Design review of the part built by this model. Coordinates are the model's own, in mm. Round coordinates to 2 decimals unless told otherwise and drop trailing zeros. Order: outer loops, then holes, each group sorted by start corner. A loop starts at its lowest first (then second) coordinate and runs counter-clockwise, first axis right, second up.
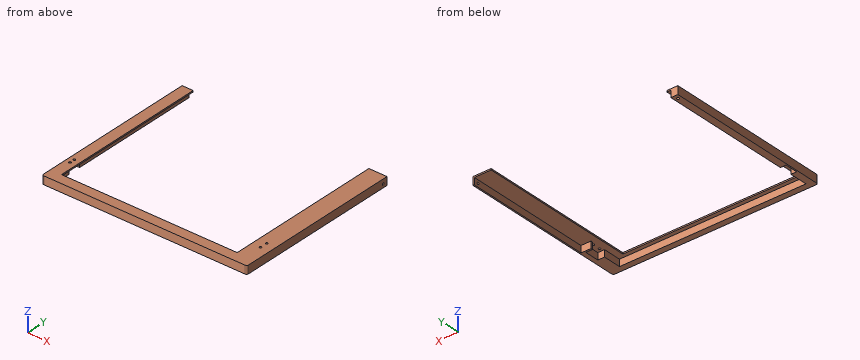
Autodesk Inventor part; units mm, degrees
ref_plane "YZ Plane" through (0, 0, 0) normal (1, 0, 0) x (0, 1, 0)
ref_plane "XZ Plane" through (0, 0, 0) normal (0, 1, 0) x (-1, 0, 0)
ref_plane "XY Plane" through (0, 0, 0) normal (0, 0, 1) x (1, 0, 0)
sketch "Boceto1" plane through (0, 0, 0) normal (0, 0, 1) x (1, 0, 0)
  circle A0 centre (100.65, -156.7) radius 1.65
  circle A1 centre (100.65, -148.3) radius 1.65
  circle A2 centre (100.65, 156.7) radius 1.65
  circle A3 centre (100.65, 148.3) radius 1.65
  line L0 (97.75, 145) -> (105.25, 145)
  line L1 (105.25, 145) -> (105.25, 160)
  line L2 (105.25, 160) -> (97.75, 160)
  line L3 (97.75, 160) -> (97.75, 180)
  line L4 (97.75, 180) -> (-109, 180)
  line L5 (-109, 160) -> (-115.3, 160)
  line L6 (-109, -160) -> (-109, -180)
  line L7 (-115.3, 146.9) -> (-109, 146.9)
  line L8 (-109, -146.9) -> (-115.3, -146.9)
  line L9 (-109, 180) -> (-109, 160)
  line L10 (-115.3, -160) -> (-109, -160)
  line L11 (-109, -180) -> (97.75, -180)
  line L12 (97.75, -180) -> (97.75, -160)
  line L13 (97.75, -160) -> (105.25, -160)
  line L14 (105.25, -160) -> (105.25, -145)
  line L15 (105.25, -145) -> (97.75, -145)
  line L16 (97.75, -145) -> (97.75, -142)
  line L17 (97.75, -142) -> (109, -142)
  line L18 (109, -142) -> (109, 142)
  line L19 (109, 142) -> (97.75, 142)
  line L20 (97.75, 142) -> (97.75, 145)
  line L21 (109, 180) -> (97.75, 180)
  line L22 (-109, -160) -> (-109, -180)
  line L23 (-109, -180) -> (-102.7, -180)
  line L24 (-109, -180) -> (109, -180)
  line L25 (109, -180) -> (109, 180)
  line L26 (109, 180) -> (-109, 180)
  line L27 (111, 142) -> (111, 180)
  line L28 (109, 182) -> (97.75, 182)
  line L29 (-109, -182) -> (-102.7, -182)
  line L30 (-111, -182) -> (111, -182)
  line L31 (111, -182) -> (111, 182)
  line L32 (111, 182) -> (-111, 182)
  circle A4 centre (-111.9, -156.3) radius 1.2
  circle A5 centre (-111.9, -150.6) radius 1.2
  circle A6 centre (-111.9, 156.3) radius 1.2
  circle A7 centre (-111.9, 150.6) radius 1.2
  line L33 (-115.3, 160) -> (-115.3, 146.9)
  line L34 (-109, 146.9) -> (-109, -146.9)
  line L35 (-115.3, -146.9) -> (-115.3, -160)
  line L36 (-109, 180) -> (-115.3, 180)
  line L37 (-109, -180) -> (-115.3, -180)
  line L38 (-115.3, 180) -> (109, 180)
  line L39 (109, 180) -> (109, -180)
  line L40 (109, -180) -> (-115.3, -180)
  line L41 (-115.3, -180) -> (-115.3, 180)
  line L42 (-117.3, 180) -> (-117.3, -182)
  line L43 (-117.3, -182) -> (109, -182)
  line L44 (-115.3, 182) -> (111, 182)
  line L45 (111, 182) -> (111, -180)
  line L46 (-117.3, 180) -> (-117.3, 182)
  line L47 (-117.3, 182) -> (-115.3, 182)
  point P0 (0, 0)
  dimension "d1" = 2
  dimension "d3" = 2
  dimension "d20" = 2
  dimension "d21" = 2
extrude "Extrusión1" add sketch "Boceto1" against normal blind 7.5 contours L0 L1 L2 L3 L21 L25 L19 L20 | L25 L24 L12 L13 L14 L15 L16 L17 | L9 L5 L41 L36 | L37 L41 L10 L6 | L7 L34 L8 L41 | L31 L30 L29 L43 L42 L46 L47 L44 L32 L28 L27
sketch "Boceto2" plane through (0, 0, 0) normal (0, 0, 1) x (1, 0, 0)
  line L0 (-117.3, -182) -> (111, -182)
  line L1 (111, -182) -> (111, 182)
  line L2 (111, 182) -> (-117.3, 182)
  line L3 (90.8, 170.8) -> (90.8, -176)
  line L4 (90.8, 170.8) -> (90.8, -176)
  line L5 (-19.4789, -176) -> (90.8, -176)
  line L6 (90.8, -176) -> (-99.7, -176)
  line L7 (-99.7, -176) -> (-99.7, 170.8)
  line L8 (-99.7, 170.8) -> (90.8, 170.8)
  line L9 (-117.3, 182) -> (-117.3, -182)
  line L10 (-105.5008, -176) -> (-99.7, -176)
  line L11 (-99.7, 170.8) -> (-105.5008, 170.8)
  line L12 (-109, 160) -> (-109, 180)
  line L13 (-109, 170.8) -> (-105, 170.8)
  line L14 (-105, 170.8) -> (-105, -176)
  point P0 (0, 0)
  dimension "d33" = 4
extrude "Extrusión2" add sketch "Boceto2" along normal blind 1.5
sketch "Boceto3" plane through (-111, -182, -7.5) normal (0, -1, 0) x (1, 0, 0)
  line L0 (222, 0) -> (-6.3, 0)
  line L1 (222, 0) -> (222, 9)
  line L2 (-6.3, 9) -> (222, 9)
  line L3 (-6.3, 0) -> (-6.3, 9)
  point P0 (111, 7.5)
extrude "Extrusión3" add sketch "Boceto3" along normal blind 5.2
sketch "Boceto5" plane through (0, 0, 1.5) normal (0, 0, 1) x (1, 0, 0)
  circle A0 centre (100.65, -156.7) radius 1.65
  circle A1 centre (100.65, -148.3) radius 1.65
  circle A2 centre (100.65, 156.7) radius 1.65
  circle A3 centre (100.65, 148.3) radius 1.65
  line L0 (97.75, 145) -> (105.25, 145)
  line L1 (105.25, 145) -> (105.25, 160)
  line L2 (105.25, 160) -> (97.75, 160)
  line L3 (97.75, 160) -> (97.75, 180)
  line L4 (97.75, 180) -> (-109, 180)
  line L5 (-109, 160) -> (-115.3, 160)
  line L6 (-109, -160) -> (-109, -180)
  line L7 (-115.3, 146.9) -> (-109, 146.9)
  line L8 (-109, -146.9) -> (-115.3, -146.9)
  line L9 (-109, 180) -> (-109, 160)
  line L10 (-115.3, -160) -> (-109, -160)
  line L11 (-109, -180) -> (97.75, -180)
  line L12 (97.75, -180) -> (97.75, -160)
  line L13 (97.75, -160) -> (105.25, -160)
  line L14 (105.25, -160) -> (105.25, -145)
  line L15 (105.25, -145) -> (97.75, -145)
  line L16 (97.75, -145) -> (97.75, -142)
  line L17 (97.75, -142) -> (109, -142)
  line L18 (109, -142) -> (109, 142)
  line L19 (109, 142) -> (97.75, 142)
  line L20 (97.75, 142) -> (97.75, 145)
  circle A4 centre (-111.9, -156.3) radius 1.2
  circle A5 centre (-111.9, -150.6) radius 1.2
  circle A6 centre (-111.9, 156.3) radius 1.2
  circle A7 centre (-111.9, 150.6) radius 1.2
  line L21 (-115.3, 160) -> (-115.3, 146.9)
  line L22 (-109, 146.9) -> (-109, -146.9)
  line L23 (-115.3, -146.9) -> (-115.3, -160)
  point P0 (0, 0)
hole "Agujero1" at (100.65, 148.3, 1.5) at (100.65, 156.7, 1.5) at (100.65, -156.7, 1.5) at (100.65, -148.3, 1.5) at (-111.9, -156.3, 1.5) at (-111.9, -150.6, 1.5) at (-111.9, 150.6, 1.5) at (-111.9, 156.3, 1.5) direction (0, 0, -1) diameter 2.4 end through all
sketch "Boceto6" plane through (0, 0, -7.5) normal (0, 0, -1) x (-1, 0, 0)
  line L0 (117.3, 182) -> (-111, 182)
  line L1 (-111, 182) -> (-111, -187.2)
  line L2 (117.3, -187.2) -> (-111, -187.2)
  line L3 (117.3, 182) -> (117.3, -187.2)
  line L4 (-97.75, 160) -> (-97.75, 180)
  line L5 (-97.75, 180) -> (109, 180)
  line L6 (109, 180) -> (109, 160)
  line L7 (109, 160) -> (115.3, 160)
  line L8 (115.3, 160) -> (115.3, 146.9)
  line L9 (115.3, 146.9) -> (109, 146.9)
  line L10 (109, 146.9) -> (109, -146.9)
  line L11 (109, -146.9) -> (115.3, -146.9)
  line L12 (115.3, -146.9) -> (115.3, -160)
  line L13 (115.3, -160) -> (109, -160)
  line L14 (109, -160) -> (109, -180)
  line L15 (109, -180) -> (-97.75, -180)
  line L16 (-97.75, -180) -> (-97.75, -160)
  line L17 (-97.75, -160) -> (-105.25, -160)
  line L18 (-105.25, -160) -> (-105.25, -145)
  line L19 (-105.25, -145) -> (-97.75, -145)
  line L20 (-97.75, -145) -> (-97.75, -142)
  line L21 (-97.75, -142) -> (-109, -142)
  line L22 (-109, -142) -> (-109, 142)
  line L23 (-109, 142) -> (-97.75, 142)
  line L24 (-97.75, 142) -> (-97.75, 145)
  line L25 (-97.75, 145) -> (-105.25, 145)
  line L26 (-105.25, 145) -> (-105.25, 160)
  line L27 (-105.25, 160) -> (-97.75, 160)
  line L28 (117.3, 182) -> (117.3, -187.2)
  line L29 (117.3, 182) -> (-111, 182)
  line L30 (-111, 182) -> (-111, -187.2)
  line L31 (117.3, -187.2) -> (-111, -187.2)
  line L32 (109.5, 160.5) -> (109.5, 180.5)
  line L33 (109.5, 180.5) -> (-98.25, 180.5)
  line L34 (-98.25, 180.5) -> (-98.25, 160.5)
  line L35 (-98.25, 160.5) -> (-105.75, 160.5)
  line L36 (-105.75, 160.5) -> (-105.75, 144.5)
  line L37 (-105.75, 144.5) -> (-98.25, 144.5)
  line L38 (-98.25, 144.5) -> (-98.25, 142.5)
  line L39 (-98.25, 142.5) -> (-109.5, 142.5)
  line L40 (-109.5, 142.5) -> (-109.5, -142.5)
  line L41 (-109.5, -142.5) -> (-98.25, -142.5)
  line L42 (-98.25, -142.5) -> (-98.25, -144.5)
  line L43 (-98.25, -144.5) -> (-105.75, -144.5)
  line L44 (-105.75, -144.5) -> (-105.75, -160.5)
  line L45 (-105.75, -160.5) -> (-98.25, -160.5)
  line L46 (-98.25, -160.5) -> (-98.25, -180.5)
  line L47 (-98.25, -180.5) -> (109.5, -180.5)
  line L48 (109.5, -180.5) -> (109.5, -160.5)
  line L49 (109.5, -160.5) -> (115.8, -160.5)
  line L50 (115.8, -160.5) -> (115.8, -146.4)
  line L51 (115.8, -146.4) -> (109.5, -146.4)
  line L52 (109.5, -146.4) -> (109.5, 146.4)
  line L53 (109.5, 146.4) -> (115.8, 146.4)
  line L54 (115.8, 146.4) -> (115.8, 160.5)
  line L55 (115.8, 160.5) -> (109.5, 160.5)
  dimension "d22" = 0.5
extrude "Extrusión4" cut sketch "Boceto6" against normal blind 7.5 contours L55 L54 L53 L52 L51 L50 L49 L48 L47 L46 L45 L44 L43 L42 L41 L40 L39 L38 L37 L36 L35 L34 L33 L32
fillet "Empalme1" radius 2 5 edges at (-117.3, 182, 0.75) (-117.3, 182, -3.75) (111, 182, -3) (111, -187.2, -3) (-117.3, -187.2, -3)
sketch "Boceto7" plane through (0, 0, -7.5) normal (0, 0, -1) x (-1, 0, 0)
  arc A0 (117.3, 7) -> (114.3, 10) centre (114.3, 7) ccw
  line L0 (114.3, 10) -> (100.3, 10)
  arc A1 (100.3, 10) -> (97.3, 7) centre (100.3, 7) ccw
  line L1 (97.3, 7) -> (97.3, -7)
  arc A2 (97.3, -7) -> (100.3, -10) centre (100.3, -7) ccw
  line L2 (100.3, -10) -> (114.3, -10)
  arc A3 (114.3, -10) -> (117.3, -7) centre (114.3, -7) ccw
  line L3 (117.3, -7) -> (117.3, 7)
  circle A4 centre (103.3, -5) radius 1
  circle A5 centre (113.3, 5) radius 1
  circle A6 centre (103.3, 5) radius 1
  circle A7 centre (113.3, -5) radius 1
  circle A8 centre (113.3, 5) radius 1
  point P0 (0, 0)
hole "Agujero2" at (-113.3, 5, -7.5) at (-113.3, -5, -7.5) direction (0, 0, 1) diameter 3 depth 6
split "Dividir4" plane through (0, 0, 0) removes the side toward (0, 1, 0)
sketch "Boceto8" plane through (111, -185.2, 1.5) normal (1, 0, 0) x (0, 0, -1)
  circle A0 centre (12.7426, 180.2) radius 1.2
  line L0 (9, 185.2) -> (0, 185.2)
  line L1 (9, 185.2) -> (9, 0)
  circle A1 centre (5.1, 190.2) radius 1.2
  line L2 (0, 185.2) -> (9, 185.2)
  line L3 (9, 365.2) -> (9, 185.2)
  line L4 (0, 365.2) -> (9, 365.2)
  line L5 (0, 365.2) -> (0, 185.2)
  line L6 (5.1, 190.2) -> (5.1, 180.2)
  point P0 (1.5, 185.2)
hole "Agujero3" at (111, -5, -3.6) direction (-1, 0, 0) diameter 2.4 depth 8 tip angle 118
properties part number "MarcoIzquierdo"
1) Take a section at A-A on y = -100. Give the boundary of the cut face in (x, z).
Results:
outline: (-117.3, -7.5) - (-109.5, -7.5) - (-109.5, 0) - (-105, 0) - (-105, 1.5) - (-117.3, 1.5) - close; (90.8, 0) - (109.5, 0) - (109.5, -7.5) - (111, -7.5) - (111, 1.5) - (90.8, 1.5) - close
2) Clearance check with flat-ended pins moving along their axes: P1, Ø3, axis at x = -113, z = -5, coming from the +Y side; P2, Ø3, axis at x = 54, z = -2.5, coming from the +Y side; P3, Ø3, axis at x = -111.9, y = -150.6, coming from the -Z side; P4, Ø2, axis at x = 103, z = -4, coming from the +Y side. State where each tip first meets the part, or that it passes through.
Results:
P1: stops at y = 0
P2: stops at y = -180.5
P3: stops at z = 0
P4: stops at y = -142.5
3) To check wall thickness, follow line 1 along X through (y, z) = (-148.3, 1); line 2 along X through (y, z) = (-150.6, 0.45); line 3 along Y through (x, z) = (-111.9, 0.8). State the ranges of each line that lie inside material, in increasing order.
Results:
line 1: x = -117.3 to -105, 90.8 to 99.45, 101.85 to 111
line 2: x = -117.3 to -113.1, -110.7 to -105, 90.8 to 111
line 3: y = -187.2 to -157.5, -155.1 to -151.8, -149.4 to 0
4) Take a section at B-B on x = -79. Give the boundary of the cut face in (y, z), plus the area to 4 significant figures.
Results:
outline: (-187.2, -7.5) - (-180.5, -7.5) - (-180.5, 0) - (-176, 0) - (-176, 1.5) - (-187.2, 1.5) - close
area: 67.05 mm2
